Geometry check sheet. Reference: the model listing, model coordinates, mm. Face numbers are marked on the shaded views. Round coordinates to 2 decimals unless told otherwise and drop trailing zeros. Order: outer loops, then holes, each group sorted by start corner. A loop starts at its lowest first (then second) coordinate and runs counter-clockwise, first axis right, second up. Notation, with made-up numbers: (21, 11.5) - (53, 11.5) arc R14 cw to (53, 33.5) - close; hole circle Ø4 at (66, 52.5). An arc over 180 degrees is marked (long way). One line per question, with ' | ' between items. Start each with the question number.
Q1. Gauge pin test, flat ends, axial feed: P1, Ø2, axis at y = -7, z = -6.5, coming from the -X side; P2, Ø6, axis at x = -24.5, z = -67.5, coming from the +Y side; P3, Ø5, axis at y = -12.5, z = -50.5, coming from the -X side. Record the tip position at first contact, or that the pin passes through.
Q2. Sectioned sample at D-D, the plane z = -129.5. Enter the section's corners in (x, y), then the cut area to 3 significant figures.
Q3. Sectioned sample at B-B, the plane z = -112.5. Enter the section's corners in (x, y).
Q4. Material ranges on line 1 along Y through (x, z) = (-42, -84); line 2 along X through (y, z) = (-5, -60.5); line 3 along X through (y, z) = (-20, -111), recorded low to high.
Q5. Sectioned sample at C-C, the plane y = 1.5. Enter the section's corners in (x, z).
Q6. Sectioned sample at A-A, the plane x = -41.5. Enter the section's corners in (y, z), then the cut area to 3 significant figures.
Q7. Mould release check, pull along X, two halves, no side actions. Record for the marked faces 1, 2, 3 and 4: +X half, -X half, draft (parallel to the pull), parting line (faces both ways), or undercut.
```python
from build123d import *

# Parameters (mm, degrees)
SKETCH2_W            = 150
SKETCH2_H            = 70
BOSS_EXTRUDE1_DEPTH  = 50
INTERSECT1_OUTLINE_W = 100
INTERSECT1_OUTLINE_H = 150
INTERSECT1_DEPTH     = 35
CUT_EXTRUDE1_DEPTH   = 153.887652053
SKETCH4_R            = 4
BOSS_EXTRUDE2_DEPTH  = 5
SKETCH8_R            = 5
CUT_EXTRUDE2_DEPTH   = 6


# Read off the part's stored shape, not the designer's step: Intersect1
with BuildPart() as part:
    # Sketch2 → Boss-Extrude1 (new, symmetric)
    with BuildSketch(Plane(origin=(0, 0, 0), x_dir=(0, 0, -1), z_dir=(1, 0, 0))):
        with Locations((65.177152604, 0)):
            Rectangle(SKETCH2_W, SKETCH2_H)
    extrude(amount=BOSS_EXTRUDE1_DEPTH, both=True)

    # Sketch1 → Cut-Revolve1 (revolve, cut)
    with BuildSketch(Plane(origin=(0, 0, 0), x_dir=(0, 0, -1), z_dir=(1, 0, 0)), mode=Mode.PRIVATE) as cut_revolve1_sk:
        with BuildLine():
            Line((140.177152604, 22.991315667), (100.177152604, 22.991315667))
            add(Edge.make_bspline(
                [(0, 0), (0.003001049, 0.012379499), (0.011197692, 0.036351162), (0.030910939, 0.072587893), (0.061826137, 0.121023529), (0.108056169, 0.183557631), (0.181890949, 0.271568579), (0.306591117, 0.401983994), (0.524430354, 0.601235581), (0.901337009, 0.902060291), (1.552737658, 1.35492318), (2.678502901, 2.03469009), (4.445764918, 2.96045388), (7.403328149, 4.31706154), (11.599431889, 5.985386832), (16.823063538, 7.814259146), (22.879973582, 9.705127394), (29.12300565, 11.472646372), (35.403551613, 13.101460315), (41.714266155, 14.60858848), (48.050573205, 16.004129586), (54.409190393, 17.293961353), (60.787889899, 18.480587367), (67.185029056, 19.563313869), (73.599488728, 20.538609835), (80.030497438, 21.398160754), (86.47762614, 22.128684831), (91.82278076, 22.603702016), (96.058091382, 22.875635683), (98.677996749, 22.971409991), (99.677383084, 22.991315667), (100.177152604, 22.991315667)],
                knots=[0, 0, 0, 0, 0, 0.000489987, 0.000979974, 0.001581787, 0.002219798, 0.003488078, 0.005411983, 0.008540376, 0.013605957, 0.022087023, 0.03601085, 0.059264391, 0.090564505, 0.147620712, 0.210220905, 0.272821133, 0.335421343, 0.398021557, 0.460621765, 0.523221981, 0.585822195, 0.648422407, 0.711022626, 0.773622837, 0.836223055, 0.89882327, 0.961423485, 0.980711742, 1, 1, 1, 1, 1], degree=4))
            Line((0, 0), (140.177152604, 0))
            Line((140.177152604, 0), (140.177152604, 22.991315667))
        make_face()
    revolve(cut_revolve1_sk.sketch.rotate(Axis((0, 0, 0), (0, 0, -1)), 90), axis=Axis((0, 0, 0), (0, 0, -1)), mode=Mode.SUBTRACT)

    # Intersect1 outline → Intersect1 (cut)
    with BuildSketch(Plane(origin=(0, 0, 0), x_dir=(1, 0, 0), z_dir=(0, 1, 0))):
        with Locations((0, 65.177152604)):
            Rectangle(INTERSECT1_OUTLINE_W, INTERSECT1_OUTLINE_H)
    extrude(amount=INTERSECT1_DEPTH, mode=Mode.SUBTRACT)

    # Sketch5 → Cut-Extrude1 (cut, through all)
    with BuildSketch(Plane(origin=(0, 0, 0), x_dir=(1, 0, 0), z_dir=(0, 1, 0))):
        Polygon((50, 86.137976919), (18.194421541, -9.822847396), (0, -21.198201401), (-18.194421541, -9.822847396), (-50, 86.137976919), (-75.365394844, 84.804131947), (-88.729692443, -46.913449713), (-13.099565549, -40.658440604), (76.90354762, -33.214709966), (74.65964276, 87.590776178), align=None)
    extrude(amount=-CUT_EXTRUDE1_DEPTH, mode=Mode.SUBTRACT)

    # Sketch4 → Boss-Extrude2 (add)
    with BuildSketch(Plane(origin=(0, 0, 0), x_dir=(1, 0, 0), z_dir=(0, 1, 0))):
        with Locations(Location((12.5, -1.822847396, 0), (0, 0, 270))):
            Circle(SKETCH4_R)
    extrude(amount=BOSS_EXTRUDE2_DEPTH)

    # Sketch8 → Cut-Extrude2 (cut)
    with BuildSketch(Plane(origin=(0, 0, 0), x_dir=(1, 0, 0), z_dir=(0, 1, 0))):
        with Locations(Location((-40, 130.177152604, 0), (0, 0, 270))):
            Circle(SKETCH8_R)
    extrude(amount=-CUT_EXTRUDE2_DEPTH, mode=Mode.SUBTRACT)


solid = part.part
```
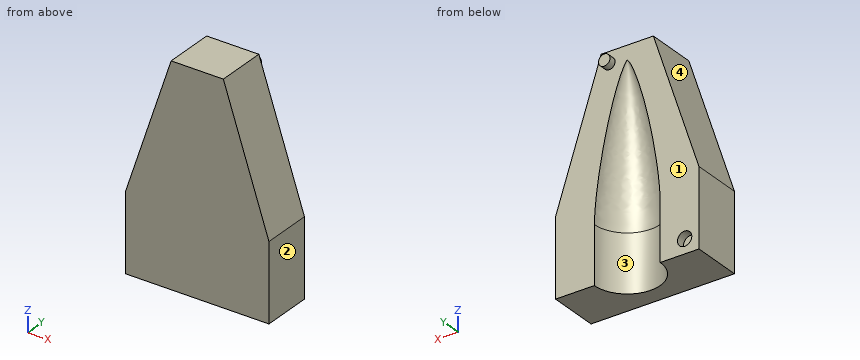
Determined:
1) P1: stops at x = -23.94 | P2: stops at y = 0 | P3: stops at x = -39.02
2) outline: (-50, -35) - (50, -35) - (50, 0) - (22.99, 0) arc R22.99 cw to (-22.99, 0) - (-35.05, 0) - (-35.05, -6) - (-44.95, -6) - (-44.95, 0) - (-50, 0) - close | area: 2,610 mm2
3) outline: (-50, -35) - (50, -35) - (50, 0) - (22.99, 0) arc R22.99 cw to (-22.99, 0) - (-50, 0) - close
4) line 1: y = -35 to 0 | line 2: x = -41.5 to -17.71, 17.71 to 41.5 | line 3: x = -50 to -11.34, 11.34 to 50
5) outline: circle Ø8 at (12.5, 1.82)
6) outline: (-35, -140.18) - (0, -140.18) - (0, -134.95) - (-6, -134.95) - (-6, -125.41) - (0, -125.41) - (0, -60.49) - (-35, -60.49) - close | area: 2,730 mm2
7) face 1: draft | face 2: +X half | face 3: undercut | face 4: -X half
